Here's how the part is built. I have some questions about the finished solid (model axes, mm). A direction names the side the tool comes from. Round coordinates to 2 decimals unless told otherwise and drop trailing zeros. Order: outer loops, then holes, each group sorted by start corner. A loop starts at its lowest first (then second) coordinate and runs counter-clockwise, first axis right, second up. Notation, with made-up numbers: M 0,-25 L 20,-25 A9 cw 20,-20 Z; hole C 80,88.5 d11. An arc over 180 degrees is marked long. Write item = value, one per line. Start each with the question number.
Item 1: I want a section at B-B, the plane x = 0. List the corners of the cut face in (y, z) for me (3 decimals).
Item 2: We'd pull the mould along Z, two halves only. Please class faces 6 (the face through (-16.95, 2.58, 5.74)), 7 (the face through (13, 0, 10)), 8 (the face through (-11, 3, 12.748)): pulls with the +Z half, pulls with the -Z half, needs draft (parallel to the pull), parting line crosses it, or undercut.
Item 3: I want a section at C-C, the plane y = 3.8. State how many separate pieces and enclosed holes the cut face has, plus the area to 3 significant figures.
Item 4: For faces 1 (the face through (47.625, 3, 46)), 2 (the face through (-23.074, 2.504, 2.624)), 3 (the face through (-9.525, 3, 31)), 4 (the face through (9.525, 3, -53)), 5 (the face through (-11, 3, -7.064)), which set-ups out of +Z, -Z, +X, -X, +Y, -Y let a thin tool reach every point of the face, with its end or its side?
Item 5: I want a section at A-A, the plane x = -11. List the corners of the cut face in (y, z) for me.
Item 6: I'm going to push flat-ended pins straight in: P1, Ø8.5, axis at x = 0, z = -45.99, coming from the +Y side; P2, Ø1.1, axis at x = -11.5, y = 3.5, coming from the -Z side; P3, Ø5.5, axis at x = -0.635, z = 4.445, coming from the -Y side; P4, Ø1, axis at y = 1.5, z = 2, coming from the -X side. Where does each tip first touch, or does it pass through?
Item 7: Please list where these lines run through material, in increasing order: L1, parallel to X at y = 1.4, z = -45 (3 decimals); L2, parallel to X at y = 2.05, z = 4.5; L3, parallel to X at y = 4, z = 39 (3 decimals).
```python
from build123d import *

# Parameters (mm, degrees)
SKETCH1_R               = 4.7625
BOSS_EXTRUDE1_DEPTH     = 5.08
SKETCH4_W               = 19.05
SKETCH4_H               = 5.08
BOSS_EXTRUDE2_DEPTH     = 5.08
SKETCH5_R               = 1.660728382
SKETCH5_R_2             = 1.651
CUT_EXTRUDE1_DEPTH      = 1.0000001
CUT_EXTRUDE1_DEPTH_BACK = 6.0800001
SKETCH6_R               = 4.7625
BOSS_EXTRUDE3_DEPTH     = 5.08
SKETCH8_R               = 4.7625
CUT_EXTRUDE2_DEPTH      = 6.0800001
SKETCH9_W               = 19.05
SKETCH9_H               = 5.08
CUT_EXTRUDE3_DEPTH      = 1.0000001
CUT_EXTRUDE3_DEPTH_BACK = 6.0800001
CUT_EXTRUDE4_DEPTH      = 1.0000001
CUT_EXTRUDE4_DEPTH_BACK = 6.0800001


with BuildPart() as part:
    # Sketch1 → Boss-Extrude1 (new body)
    with BuildSketch(Plane(origin=(0, 0, 0), x_dir=(1, 0, 0), z_dir=(0, 1, 0))):
        with BuildLine():
            Line((-9.525, 53.975), (9.525, 53.975))
            Line((9.525, 53.975), (9.525, 51.435))
            add(Edge.make_bspline(
                [(9.525, 51.435), (9.525, 51.21454564), (27.819109584, -48.895), (60.325, -48.895)],
                knots=[0, 0, 0, 0, 1, 1, 1, 1], degree=3))
            Line((60.325, -48.895), (-9.525, -48.895))
            Line((-9.525, -48.895), (-9.525, 53.975))
        make_face()
        with Locations((0, 45.9867)):
            Circle(SKETCH1_R, mode=Mode.SUBTRACT)
    extrude(amount=BOSS_EXTRUDE1_DEPTH)

    # Sketch4 → Boss-Extrude2 (add)
    with BuildSketch(Plane(origin=(0, 5.08, 0), x_dir=(1, 0, 0), z_dir=(0, 1, 0))):
        with Locations((50.8, -51.435)):
            Rectangle(SKETCH4_W, SKETCH4_H)
    extrude(amount=-BOSS_EXTRUDE2_DEPTH)

    # Sketch5 → Cut-Extrude1 (cut, two sides)
    with BuildSketch(Plane.XZ) as cut_extrude1_sk:
        with Locations((-0.635, 4.445)):
            Circle(SKETCH5_R)
        with Locations((37.465, 40.005)):
            Circle(SKETCH5_R_2)
    extrude(amount=CUT_EXTRUDE1_DEPTH, mode=Mode.SUBTRACT)
    extrude(cut_extrude1_sk.sketch, amount=-CUT_EXTRUDE1_DEPTH_BACK, mode=Mode.SUBTRACT)

    # Sketch6 → Boss-Extrude3 (add)
    with BuildSketch(Plane.XZ):
        with BuildLine():
            Line((-13.170662, 12.74826), (-9.525, 12.74826))
            Line((-9.525, 12.74826), (-9.525, 12.053013747))
            ThreePointArc((-9.525, 12.053013747), (-3.264662, 2.84226), (-9.525, -6.368493747))
            Line((-9.525, -6.368493747), (-9.525, -7.06374))
            Line((-9.525, -7.06374), (-13.170662, -7.06374))
            ThreePointArc((-13.170662, -7.06374), (-23.076662, 2.84226), (-13.170662, 12.74826))
        make_face()
        with Locations((-13.170662, 2.84226)):
            Circle(SKETCH6_R, mode=Mode.SUBTRACT)
    extrude(amount=-BOSS_EXTRUDE3_DEPTH)

    # Sketch8 → Cut-Extrude2 (cut, through all)
    with BuildSketch(Plane(origin=(0, 5.08, 0), x_dir=(1, 0, 0), z_dir=(0, 1, 0))):
        with Locations((-13.170662, -2.84226)):
            Circle(SKETCH8_R)
    extrude(amount=-CUT_EXTRUDE2_DEPTH, mode=Mode.SUBTRACT)

    # Sketch9 → Cut-Extrude3 (cut, two sides)
    with BuildSketch(Plane.XZ) as cut_extrude3_sk:
        with Locations((50.8, 51.435)):
            Rectangle(SKETCH9_W, SKETCH9_H)
    extrude(amount=CUT_EXTRUDE3_DEPTH, mode=Mode.SUBTRACT)
    extrude(cut_extrude3_sk.sketch, amount=-CUT_EXTRUDE3_DEPTH_BACK, mode=Mode.SUBTRACT)

    # Sketch10 → Cut-Extrude4 (cut, two sides)
    with BuildSketch(Plane.XZ) as cut_extrude4_sk:
        with BuildLine():
            Line((47.625, 43.646486826), (47.625, 48.895))
            Line((47.625, 48.895), (60.325, 48.895))
            add(Edge.make_bspline(
                [(60.325, 48.895), (55.814379896, 48.895), (51.577410685, 46.967369191), (47.625, 43.646486826)],
                knots=[0, 0, 0, 0, 0.138763161, 0.138763161, 0.138763161, 0.138763161], degree=3))
        make_face()
    extrude(amount=CUT_EXTRUDE4_DEPTH, mode=Mode.SUBTRACT)
    extrude(cut_extrude4_sk.sketch, amount=-CUT_EXTRUDE4_DEPTH_BACK, mode=Mode.SUBTRACT)


solid = part.part
```
Filled in:
q1.outline = M 0,-53.975 L 5.08,-53.975 L 5.08,-50.749 L 0,-50.749 Z; M 0,-41.224 L 5.08,-41.224 L 5.08,2.91 L 0,2.91 Z; M 0,5.98 L 5.08,5.98 L 5.08,48.895 L 0,48.895 Z
q2.face_6 = undercut
q2.face_7 = needs draft
q2.face_8 = pulls with the +Z half
q3.separate_pieces = 1
q3.enclosed_holes = 4
q3.area = 3,570 mm^2
q4.face_1 = +Z, -Z, +X, +Y, -Y
q4.face_2 = -X, +Y, -Y
q4.face_3 = +Z, -X, +Y, -Y
q4.face_4 = -Z, +X, +Y, -Y
q4.face_5 = -Z, -X, +Y, -Y
q5.outline = M 0,-7.06 L 5.08,-7.06 L 5.08,-1.4 L 0,-1.4 Z; M 0,7.08 L 5.08,7.08 L 5.08,12.75 L 0,12.75 Z
q6.P1 = through
q6.P2 = -7.06
q6.P3 = 0
q6.P4 = -23.07
q7.L1 = -9.525 to -4.659, 4.659 to 10.803
q7.L2 = -22.94 to -17.64, -8.71 to -2.29, 1.02 to 24.77
q7.L3 = -9.525 to 36.155, 38.775 to 42.996
